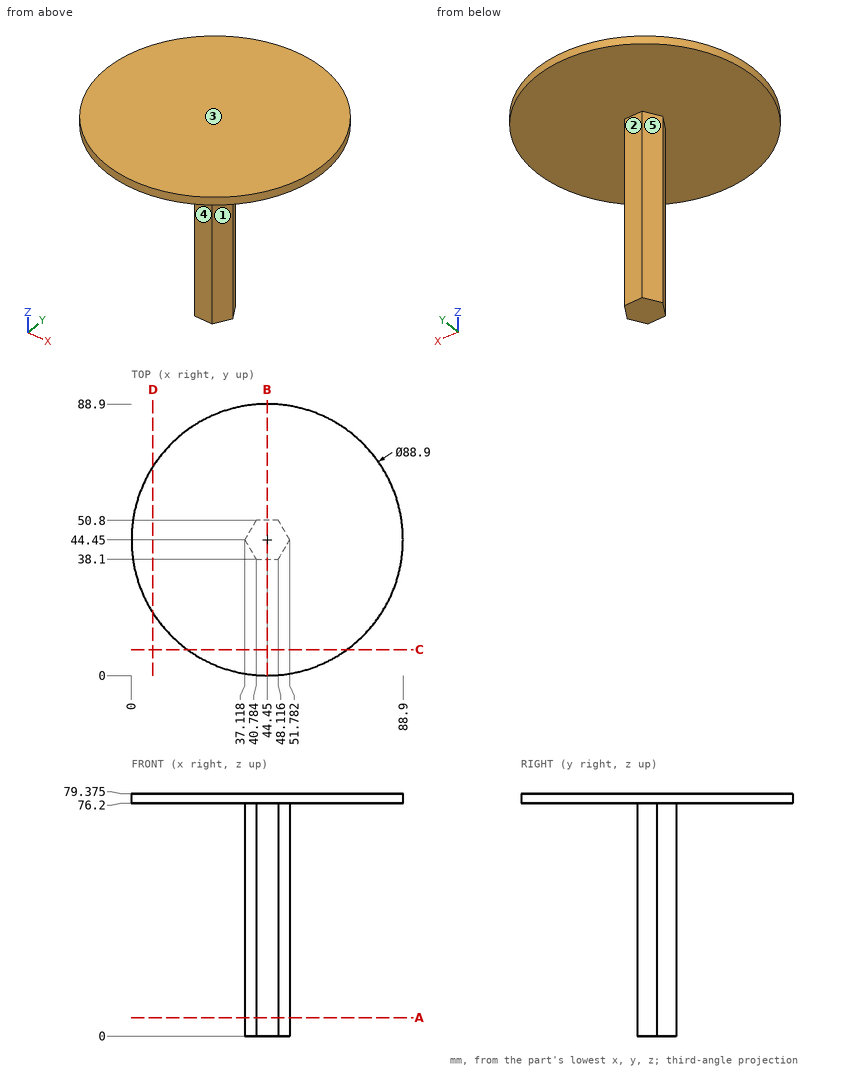
Source: three-view drawing plus pictorial views. Frame: mm from the lowest corner of the part. A direction names the side the tool comes from. Round coordinates to 2 decimals unless told otherwise and drop trailing zeros. Loops run counter-clockwise (first coordinate to the right, second up) from the corner with the lowest first, then second, coordinate; pieces in that order, holes last. Notation, with made-up numbers: (64, 76.25) - (110, 76.25) arc R29 ccw to (110, 114.25) - close; hole circle Ø3 at (73, -21). An arc over 180 degrees is marked (long way). Write item = value, one per line. Start each with the question number.
Item 1: Reachability of the marked faces 1, 2, 3, 4 and 5 from +Z, -Z, +X, -X, +Y, -Y: full face, straight path, thin tool, end or side. Return the list, or none.
Item 2: Material intervals for line 1 (Z direction, x = 72.5, y = 64) (1 decimal); line 2 (Y direction, x = 44, z = 18); line 3 (X direction, y = 42, z = 48), sorted ascending.
Item 3: Section query C-C on y = 8.5. Output: boundary loops of the cut face in (x, z) (1 decimal).
Item 4: Section query D-D on x = 7. Output: boundary loops of the cut face in (y, z) (1 decimal).
Item 5: Section query B-B on x = 44.45. Output: boundary loops of the cut face in (y, z) (1 decimal).
Item 6: First-contact query: pin 1 Ø1 at (x, y) = (61, 35.5) entering from -Z; pin 2 Ø6 at (x, z) = (46, 40) entering from -Y; pin 3 Ø6 at (x, z) = (44.5, 41) entering from +Y. Flat tips, straight axial feed; report the tip coordinate or a pass-through.
Item 7: Section query A-A on z = 6. Output: boundary loops of the cut face in (x, y).
Results list:
q1.face_1 = -Z, +X, -Y
q1.face_2 = -Z, +X, -X, +Y
q1.face_3 = +Z, +X, -X, +Y, -Y
q1.face_4 = -Z, +X, -X, -Y
q1.face_5 = -Z, -X, +Y
q2.line_1 = 76.2 to 79.4
q2.line_2 = 38.1 to 50.8
q2.line_3 = 38.53 to 50.37
q3.outline = (18.3, 76.2) - (70.6, 76.2) - (70.6, 79.4) - (18.3, 79.4) - close
q4.outline = (20.5, 76.2) - (68.4, 76.2) - (68.4, 79.4) - (20.5, 79.4) - close
q5.outline = (0, 76.2) - (38.1, 76.2) - (38.1, 0) - (50.8, 0) - (50.8, 76.2) - (88.9, 76.2) - (88.9, 79.4) - (0, 79.4) - close
q6.pin_1 = 76.2
q6.pin_2 = 38.1
q6.pin_3 = 50.8
q7.outline = (37.12, 44.45) - (40.78, 38.1) - (48.12, 38.1) - (51.78, 44.45) - (48.12, 50.8) - (40.78, 50.8) - close
